Model file for the job. Use its own axes, mm. A direction names the side the tool comes from. Give positions to 0.01 mm unless a question says otherwise; leave off trailing zeros. Loops run counter-clockwise (first coordinate to the right, second up) from the corner with the lowest first, then second, coordinate; pieces in that order, holes last. Notation, with made-up numbers: M 25.25,33 L 58.25,33 A35 cw 58.25,67 Z; hole C -7,-25 d10. An arc over 180 degrees is marked long. Use CSV: the item, a comma, the result in double quotes. Start each with the question number.
(1) Wall check: line 1 along Y through (x, z) = (-1.55, 1.25); line 2 along X through (y, z) = (-0.3, 0.55); line 3 along X through (y, z) = (-1.4, 1.4). Give the ranges that are in metal, low to high. Write a range as from..to.
(2) Slice it at C-C on y = -2. List the corners of the cut face in (x, z).
(3) Tool access for faces 5 (the face through (0.3, -0.2, 0)), 6 (the face through (0, -1, 1)), 7 (the face through (-3, 0, 1)): list every direction of +Z, -Z, +X, -X, +Y, -Y with a clear straight run to the whole face (end or side of a thin tool).
(4) Flat gauge pins, fed straight in: P1, Ø1.2, axis at x = -1.5, z = 1, coming from the +Y side; P2, Ø1, axis at y = -1.5, z = 1.5, coming from the -X side; P3, Ø1.5, axis at x = 4, z = 0.5, coming from the -Y side. Where does each tip first touch, or does it go through?
(5) Slice it at B-B on z = 0.4. List the corners of the cut face in (x, y), and give its area (3 significant figures).
(6) Slice it at D-D on z = 1.25. List the corners of the cut face in (x, y), and give its area (3 significant figures).
(7) Two-plate mould, pull along Y, no slides. Class faces 1 (the face through (0.876, -1.013, 1.264)), 2 (the face through (0.3, -0.2, 2.5)), 3 (the face through (2.926, 0.492, 0.274)), 4 (the face through (3.22, -0.56, 1.23)): pulls with the +Y half, pulls with the -Y half, needs draft (parallel to the pull), parting line crosses it, or undercut.
(8) Slice it at A-A on x = -3.5. List the corners of the cut face in (y, z).
```python
from build123d import *

# Parameters (mm, degrees)
BOSS_EXTRUDE1_DEPTH = 2.5
SKETCH2_R           = 1
CUT_EXTRUDE1_DEPTH  = 5
SKETCH3_R           = 1
CUT_EXTRUDE2_DEPTH  = 5


with BuildPart() as part:
    # Sketch1 → Boss-Extrude1 (new body)
    with BuildSketch(Plane.XY):
        Polygon((-5, 0), (0, 0), (3.830222216, 3.213938048), (5.465982834, 1.323359513), (0.909480399, -2.5), (-5, -2.5), align=None)
    extrude(amount=BOSS_EXTRUDE1_DEPTH)

    # Sketch2 → Cut-Extrude1 (cut)
    with BuildSketch(Plane(origin=(3.780724263, 3.271146765, 0), x_dir=(0, 0, -1), z_dir=(0.7562314141303861, 0.6543042474891606, 0))):
        with Locations(Location((-1.25, -1.325649749, 0), (0, 0, 90))):
            Circle(SKETCH2_R)
    extrude(amount=-CUT_EXTRUDE1_DEPTH, mode=Mode.SUBTRACT)

    # Sketch3 → Cut-Extrude2 (cut)
    with BuildSketch(Plane.ZY.offset(5)):
        with Locations((1.25, -1.25)):
            Circle(SKETCH3_R)
    extrude(amount=-CUT_EXTRUDE2_DEPTH, mode=Mode.SUBTRACT)


solid = part.part
```
Reply:
1,line 1,"y = -2.5..-2.25, -0.25..0"
1,line 2,"x = -5..0.59, 2.77..3.53"
1,line 3,"x = 0..1.21, 1.92..2.22"
2,outline,"M -5,0 L 1.51,0 L 1.51,2.5 L -5,2.5 L -5,1.91 L 0,1.91 L 0,0.59 L -5,0.59 Z"
3,face 5,"-Z, +X, -X, +Y, -Y"
3,face 6,"-X"
3,face 7,"+Z, -Z, -X, +Y"
4,P1,"stops at y = 0"
4,P2,"stops at x = 0"
4,P3,"stops at y = -0.54"
5,outline,"M -5,-2.5 L 0.91,-2.5 L 5.47,1.32 L 4.99,1.87 L 1.21,-1.4 L 0.52,-0.6 L 4.3,2.67 L 3.83,3.21 L 0,0 L -5,0 L -5,-0.72 L 0,-0.72 L 0,-1.78 L -5,-1.78 Z"
5,area,"16.8 mm^2"
6,outline,"M -5,-2.5 L 0.91,-2.5 L 5.47,1.32 L 5.3,1.51 L 1.52,-1.76 L 0.21,-0.25 L 3.99,3.02 L 3.83,3.21 L 0,0 L -5,0 L -5,-0.25 L 0,-0.25 L 0,-2.25 L -5,-2.25 Z"
6,area,"7.32 mm^2"
7,face 1,"undercut"
7,face 2,"needs draft"
7,face 3,"undercut"
7,face 4,"pulls with the -Y half"
8,outline,"M -2.5,0 L 0,0 L 0,2.5 L -2.5,2.5 Z; hole C -1.25,1.25 d2"
